from build123d import *

# Parameters (mm, degrees)
F0_W          = 10.16
F0_H          = 6.35
F0_R          = 1.98
F0_W_2        = 8
F0_H_2        = 1.57
F0_W_3        = 71.65
F0_H_3        = 1.6
F0_W_4        = 11.65
F1_DEPTH      = 1.57
F2_DEPTH      = 11.25
F3_R          = 1.5
F4_DEPTH      = 6.43
F0_W_5        = 0.94
F0_H_4        = 158.75
F5_DEPTH      = 3.81
F5_DEPTH_BACK = 40.64
F6_W          = 44.45
F6_H          = 158.75
F6_W_2        = 40.45
F6_H_2        = 154.75
F7_DEPTH      = 2
F8_R          = 0.99999
F9_W          = 30
F9_H          = 15
F10_DEPTH     = 20
F9_W_2        = 25
F9_H_2        = 35
F11_DEPTH     = 25
F9_H_3        = 18
F12_DEPTH     = 30
F9_W_3        = 38
F9_H_4        = 25
F13_DEPTH     = 23
F14_SIZE      = 5
F15_W         = 4
F15_H         = 1.6
F16_DEPTH     = 2
F17_DEPTH     = 7.9


# Not quite as in the source:
# - a fillet or chamfer is up to 0.001 mm smaller than in the source, because OpenCascade refuses the exact size


with BuildPart() as f1:
    # F0 (on Right) → F1 (new body)
    with BuildSketch(Plane.YZ):
        with Locations((5.08, 206.375)):
            Rectangle(F0_W, F0_H)
        with BuildLine():
            Line((0, 203.2), (0, 209.55))
            Line((0, 209.55), (-22.86, 209.55))
            Line((-22.86, 209.55), (-22.86, 205.18))
            ThreePointArc((-22.86, 205.18), (-21.4599285733, 204.6000714267), (-20.88, 203.2))
            Line((-20.88, 203.2), (0, 203.2))
        make_face()
        with BuildLine():
            Line((-22.86, 205.18), (-22.86, 209.55))
            Line((-22.86, 209.55), (-154.94, 209.55))
            Line((-154.94, 209.55), (-154.94, 205.18))
            ThreePointArc((-154.94, 205.18), (-153.5399285733, 204.6000714267), (-152.96, 203.2))
            Line((-152.96, 203.2), (-24.84, 203.2))
            ThreePointArc((-24.84, 203.2), (-24.2600714267, 204.6000714267), (-22.86, 205.18))
        make_face()
        with BuildLine():
            Line((-154.94, 205.18), (-154.94, 209.55))
            Line((-154.94, 209.55), (-160.02, 209.55))
            Line((-160.02, 209.55), (-160.02, 203.2))
            Line((-160.02, 203.2), (-156.92, 203.2))
            ThreePointArc((-156.92, 203.2), (-156.3400714267, 204.6000714267), (-154.94, 205.18))
        make_face()
        with BuildLine():
            Line((0, 47.7), (0, 203.2))
            Line((0, 203.2), (-20.88, 203.2))
            ThreePointArc((-20.88, 203.2), (-22.86, 201.22), (-24.84, 203.2))
            Line((-24.84, 203.2), (-152.96, 203.2))
            ThreePointArc((-152.96, 203.2), (-154.94, 201.22), (-156.92, 203.2))
            Line((-156.92, 203.2), (-160.02, 203.2))
            Line((-160.02, 203.2), (-160.02, 39.37))
            Line((-160.02, 39.37), (0, 39.37))
            Line((0, 39.37), (0, 43.74))
            ThreePointArc((0, 43.74), (-1.98, 45.72), (0, 47.7))
        make_face()
        with Locations((-154.94, 45.72)):
            Circle(F0_R, mode=Mode.SUBTRACT)
        Polygon((-121.44, 51.04), (-46.94, 51.04), (-32.44, 51.04), (-32.44, 43.54), (-46.94, 43.54), (-121.44, 43.54), align=None, mode=Mode.SUBTRACT)
        with Locations((-27.14, 47.29)):
            Rectangle(F0_W_2, F0_H_2, mode=Mode.SUBTRACT)
        with BuildLine():
            Line((10.16, 45.72), (10.16, 203.2))
            Line((10.16, 203.2), (0, 203.2))
            Line((0, 203.2), (0, 47.7))
            ThreePointArc((0, 47.7), (1.4000714267, 47.1200714267), (1.98, 45.72))
            Line((1.98, 45.72), (10.16, 45.72))
        make_face()
        with BuildLine():
            Line((10.16, 39.37), (10.16, 45.72))
            Line((10.16, 45.72), (1.98, 45.72))
            ThreePointArc((1.98, 45.72), (1.4000714267, 44.3199285733), (0, 43.74))
            Line((0, 43.74), (0, 39.37))
            Line((0, 39.37), (10.16, 39.37))
        make_face()
        Polygon((-32.44, 51.04), (-46.94, 51.04), (-121.44, 51.04), (-121.44, 43.54), (-46.94, 43.54), (-32.44, 43.54), align=None)
        with Locations((-83.615, 47.29)):
            Rectangle(F0_W_3, F0_H_3, mode=Mode.SUBTRACT)
        with Locations((-40.265, 47.29)):
            Rectangle(F0_W_4, F0_H_3, mode=Mode.SUBTRACT)
        with Locations((-40.265, 47.29)):
            Rectangle(F0_W_4, F0_H_3)
        with Locations((-83.615, 47.29)):
            Rectangle(F0_W_3, F0_H_3)
        with Locations((-27.14, 47.29)):
            Rectangle(F0_W_2, F0_H_2)
    extrude(amount=F1_DEPTH)

    # F0 (on Right) → F2 (join)
    with BuildSketch(Plane.YZ):
        Polygon((-32.44, 51.04), (-46.94, 51.04), (-121.44, 51.04), (-121.44, 43.54), (-46.94, 43.54), (-32.44, 43.54), align=None)
        with Locations((-83.615, 47.29)):
            Rectangle(F0_W_3, F0_H_3, mode=Mode.SUBTRACT)
        with Locations((-40.265, 47.29)):
            Rectangle(F0_W_4, F0_H_3, mode=Mode.SUBTRACT)
    extrude(amount=-F2_DEPTH)

    # F3 (on face) → F4 (join)
    with BuildSketch(Plane.YZ.offset(1.57)):
        Polygon((-154.94, 200.2), (-152.3419237886, 201.7), (-152.3419237886, 204.7), (-154.94, 206.2), (-157.5380762114, 204.7), (-157.5380762114, 201.7), align=None)
        with Locations((-154.94, 203.2)):
            Circle(F3_R, mode=Mode.SUBTRACT)
        Polygon((-154.94, 42.72), (-152.3419237886, 44.22), (-152.3419237886, 47.22), (-154.94, 48.72), (-157.5380762114, 47.22), (-157.5380762114, 44.22), align=None)
        with Locations((-154.94, 45.72)):
            Circle(F3_R, mode=Mode.SUBTRACT)
        Polygon((0, 42.72), (2.5980762114, 44.22), (2.5980762114, 47.22), (0, 48.72), (-2.5980762114, 47.22), (-2.5980762114, 44.22), align=None)
        with Locations((0, 45.72)):
            Circle(F3_R, mode=Mode.SUBTRACT)
        Polygon((-22.86, 200.2), (-20.2619237886, 201.7), (-20.2619237886, 204.7), (-22.86, 206.2), (-25.4580762114, 204.7), (-25.4580762114, 201.7), align=None)
        with Locations((-22.86, 203.2)):
            Circle(F3_R, mode=Mode.SUBTRACT)
    extrude(amount=F4_DEPTH)



with BuildPart() as f5:
    # F0 (on Right) → F5 (new body, two sides)
    with BuildSketch(Plane.YZ) as f5_sk:
        with Locations((12.74, 132.615)):
            Rectangle(F0_W_5, F0_H_4)
    extrude(amount=F5_DEPTH)
    extrude(f5_sk.sketch, amount=-F5_DEPTH_BACK)

    # F6 (on face) → F7 (join)
    with BuildSketch(Plane(origin=(0, 13.21, 0), x_dir=(-1, 0, 0), z_dir=(0, 1, 0))):
        with Locations((18.415, 132.615)):
            Rectangle(F6_W, F6_H)
        with Locations((18.415, 132.615)):
            Rectangle(F6_W_2, F6_H_2, mode=Mode.SUBTRACT)
    extrude(amount=F7_DEPTH)

    # F8 (radius 1 in the source; OpenCascade refuses exactly that, so slightly less here)
    f8_edges = [f5.edges().sort_by_distance(p)[0] for p in [
        (1.81, 15.21, 132.615),
        (-18.415, 15.21, 209.99),
        (-38.64, 15.21, 132.615),
        (-18.415, 15.21, 55.24),
        (-18.415, 15.21, 53.24),
        (-40.64, 15.21, 132.615),
        (3.81, 15.21, 132.615),
        (-18.415, 15.21, 211.99),
    ]]
    fillet(f8_edges, radius=F8_R)


with BuildPart() as f1_1:
    add(f1.part)

    add(f5.part)  # F10 merges F5
    # F9 (on face) → F10 (join)
    with BuildSketch(Plane.XZ.offset(-12.27)):
        with Locations((-15, 184.49)):
            Rectangle(F9_W, F9_H)
    extrude(amount=F10_DEPTH)

    # F9 (on face) → F11 (join)
    with BuildSketch(Plane.XZ.offset(-12.27)):
        with Locations((-12.5, 149.49)):
            Rectangle(F9_W_2, F9_H_2)
    extrude(amount=F11_DEPTH)

    # F9 (on face) → F12 (join)
    with BuildSketch(Plane.XZ.offset(-12.27)):
        with Locations((-15, 112.99)):
            Rectangle(F9_W, F9_H_3)
    extrude(amount=F12_DEPTH)

    # F9 (on face) → F13 (join)
    with BuildSketch(Plane.XZ.offset(-12.27)):
        with Locations((-19, 85.49)):
            Rectangle(F9_W_3, F9_H_4)
    extrude(amount=F13_DEPTH)

    # F14
    f14_edges = [f1_1.edges().sort_by_distance(p)[0] for p in [
        (-25, -12.73, 149.49),
    ]]
    chamfer(f14_edges, length=F14_SIZE)

    # F15 (on face) → F16 (cut)
    with BuildSketch(Plane(origin=(0, -46.09, 0), x_dir=(-1, 0, 0), z_dir=(0, 1, 0))):
        with Locations((2, 47.29)):
            Rectangle(F15_W, F15_H)
    extrude(amount=-F16_DEPTH, mode=Mode.SUBTRACT)

    # F0 (on Right) → F17 (join)
    with BuildSketch(Plane.YZ):
        with Locations((-27.14, 47.29)):
            Rectangle(F0_W_2, F0_H_2)
    extrude(amount=-F17_DEPTH)


solid = f1_1.part
Design review of the part built by this model. Coordinates are the model's own, in mm. A direction names the side the tool comes from. Give positions to 0.01 mm unless a question says otherwise; leave off trailing zeros. Order: outer loops, then holes, each group sorted by start corner. A loop starts at its lowest first (then second) coordinate and runs counter-clockwise, first axis right, second up.
1. To check wall thickness, follow L1, parallel to Z at x = 5.5, y = -154.94; L2, parallel to Z at x = -9.5, y = -39; L3, parallel to Z at x = 0.7, y = -154.94. State the ranges of each line that lie inside material, in increasing order.
Solution:
L1: z = 42.72 to 44.22, 47.22 to 48.72, 200.2 to 201.7, 204.7 to 206.2
L2: z = 43.54 to 46.49, 48.09 to 51.04
L3: z = 39.37 to 43.74, 47.7 to 201.22, 205.18 to 209.55
2. For pin 1 Ø1.5 at (x, z) = (5.5, 203) entering from -Y; pin 2 Ø2 at (x, z) = (-4, 49) entering from +Y; pin 3 Ø4 at (x, z) = (-10.5, 114.5) entering from +Y; pin 4 Ø1.5 at (x, y) = (-13, -50.5) entering from -Z, all flat-tipped, find the tip position at first contact; note any pin that passes through.
Solution:
pin 1: stops at y = -157.54
pin 2: stops at y = -23.14
pin 3: stops at y = 13.21
pin 4: passes through
3. Mouldability with a two-part tool opening along X and no side actions: class faces 1 (the flat face through (1.57, -76, 126)), 2 (the flat face through (-11.25, -78, 49)), 3 (the flat face through (-18, 13.21, 132)), 4 (the flat face through (-15, -3, 103.99)) as +X half, -X half, draft (parallel to the pull), parting line (faces both ways), or undercut.
Solution:
face 1: +X half
face 2: -X half
face 3: undercut
face 4: draft
4. Tool access review of faces 5 (the flat face through (-15, -17.73, 113)), 6 (the flat face through (-19, -10.73, 86)), 7 (the cylindrical face through (0.774, -156.918, 45.807)), 8 (the flat face through (-22.465, -10.265, 149.245)), 9 (the flat face through (-13, 0, 166.99)): name each direction out of +Z, -Z, +X, -X, +Y, -Y from which nothing blocks a thin tool from reaching the whole face with its end or side.
Solution:
face 5: +Z, -Z, -X, -Y
face 6: -Z, -X, -Y
face 7: -X
face 8: +Z, -X, -Y
face 9: -X, -Y
5. Add section A-A, the plane y = -83.5. State the section outline as (x, z) points, then the cut area to 3 significant figures.
Solution:
outline: (-11.25, 43.54) - (0, 43.54) - (0, 39.37) - (1.57, 39.37) - (1.57, 209.55) - (0, 209.55) - (0, 51.04) - (-11.25, 51.04) - (-11.25, 48.09) - (0, 48.09) - (0, 46.49) - (-11.25, 46.49) - close
area: 334 mm2
